from build123d import *

# Parameters (mm, degrees)
SKETCH1_R           = 10
BOSS_EXTRUDE1_DEPTH = 2.6


with BuildPart() as part:
    # Sketch1 → Boss-Extrude1 (new body)
    with BuildSketch(Plane(origin=(0, 0, 0), x_dir=(1, 0, 0), z_dir=(0, 1, 0))):
        with Locations((-44.462988446, 0)):
            Circle(SKETCH1_R)
        with BuildLine():
            Line((-29.565238745, 11.34310087), (-45.335497693, 9.961863662))
            ThreePointArc((-45.335497693, 9.961863662), (-37.707438597, 7.373096109), (-34.462988446, 0))
            ThreePointArc((-34.462988446, 0), (-37.391920635, -7.071067812), (-44.462988446, -10))
            Line((-44.462988446, -10), (-29.565238745, -10))
            Line((-29.565238745, -10), (-29.565238745, 11.34310087))
        make_face()
        with BuildLine():
            Line((-29.565238745, -10), (2.323097165, -10))
            ThreePointArc((2.323097165, -10), (3.374896218, 0.688910471), (2.015736466, 11.34310087))
            Line((2.015736466, 11.34310087), (-29.565238745, 11.34310087))
            Line((-29.565238745, 11.34310087), (-29.565238745, -10))
        make_face()
    extrude(amount=BOSS_EXTRUDE1_DEPTH)


solid = part.part
For this review, take the finished solid that the model builds, in its own axes (mm). Coordinates: 2 decimals unless noted, no trailing zeros. Write each loop counter-clockwise with the first axis right and the second up, starting at its lowest first coordinate (ties: lowest second). Pieces come first, ordered by that corner, then holes. Notation, with made-up numbers: (41, 79) -> (59, 79) arc R19 cw to (59, 106) -> close; hole circle Ø7 at (-19.5, 75). An arc over 180 degrees is marked (long way). Write each question's results on one line, items separated by ' | '. Start each with the question number.
1) Consider section A-A (y = 1.55). Write out the cut boundary in (x, z), plus the area to 3 significant figures.
2) Wall thickness on L1, parallel to X at y = 2.4, z = 0; L2, parallel to X at y = 1.2, z = 1.25; L3, parallel to Z at x = -47, y = 0.55: over which ranges is each line inside the solid? List them lowest first. Write a range as [from, to].
3) Consider section B-B (x = -43.5). Write out the cut boundary in (y, z), plus the area to 3 significant figures.
4) Consider section C-C (z = -9). Write out the cut boundary in (x, y).
5) Insertion check: pin 1 (1.5 mm diameter, centred on y = 2, z = -4, fed in from -X); pin 2 (1.5 mm diameter, centred on y = 1, z = 4, fed in from +X). Each pin has a flat end and moves straight along its axis. Give the tip position at first contact, or say it passes through.
Geometry says:
1) outline: (-45.34, -9.96) -> (-29.57, -11.34) -> (2.02, -11.34) arc R47.84 ccw to (2.32, 10) -> (-44.46, 10) arc R10 ccw to start | area: 1,160 mm^2
2) L1: [-54.46, 3.38] | L2: [-54.38, 3.36] | L3: [-9.67, 9.67]
3) outline: (0, -10.12) -> (2.6, -10.12) -> (2.6, 10) -> (0, 10) -> close | area: 52.3 mm^2
4) outline: (-48.82, 0) -> (2.53, 0) -> (2.53, 2.6) -> (-48.82, 2.6) -> close
5) pin 1: x = -53.92 | pin 2: x = 3.27
